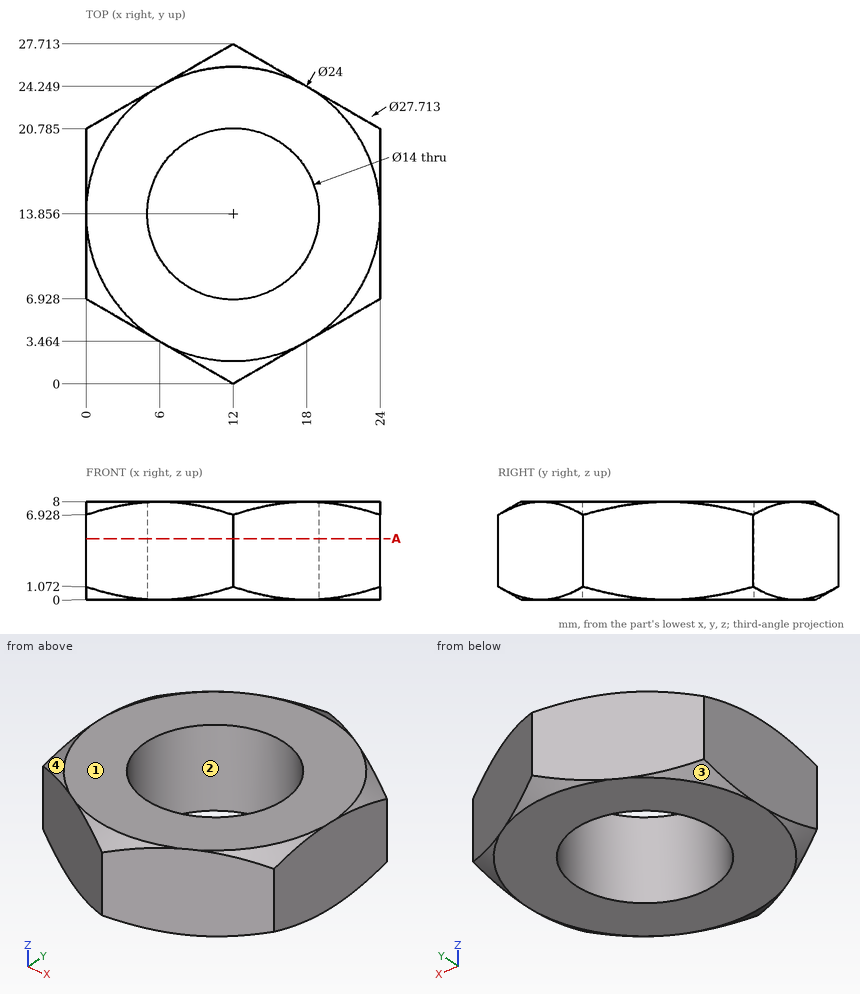
Answer from the drawing. Dimensions are ordinates in mm from the lowest x, y and z of the part. Give positions to 0.01 mm unless a question says otherwise; leave off trailing zeros. Write each loop counter-clockwise with the first axis right and the second up, starting at its lowest first coordinate (ties: lowest second). Pieces come first, ordered by that corner, then holes. Notation, with made-up numbers: (56.25, 0) -> (98.25, 0) arc R20 cw to (98.25, 22) -> close; hole circle Ø1 at (0.25, -6.75). An arc over 180 degrees is marked (long way). Use a Markdown table: item, result.
(1) Flat-ended cylindrical pins translate along their axes: P1, Ø1, axis at x = 21.5, z = 1.5, coming from the +Y side; P2, Ø1.5, axis at x = 14, z = 5, coming from the -Y side. Find the tip coordinate at first contact, or state that the pin passes through.
Return value:
| item | result |
|---|---|
| P1 | y = 22.52 |
| P2 | y = 0.72 |
(2) Find the intervals of material crossed by probe 1 along X at (y, z) = (18, 2); probe 2 along X at (y, z) = (9.25, 3.25); probe 3 along Y at (x, z) = (17, 2) (1 decimal), in increasing order. Write a range as from..to.
Return value:
| item | result |
|---|---|
| probe 1 | 0..6.36, 17.64..24 |
| probe 2 | 0..6.73, 17.27..24 |
| probe 3 | 2.9..9, 18.8..24.8 |
(3) Determine the mould class of the marked faces 1, 2, 3 and 4 for opening direction Y: released by +Y, released by -Y, zero draft, split by the parting line, or undercut.
Return value:
| item | result |
|---|---|
| face 1 | zero draft |
| face 2 | undercut |
| face 3 | released by +Y |
| face 4 | released by -Y |
(4) Section A-A, the plane z = 5 is taken. Determine the outline of the cut face in (x, y) (1 decimal).
Return value:
| item | result |
|---|---|
| outline | (0, 6.9) -> (12, 0) -> (24, 6.9) -> (24, 20.8) -> (12, 27.7) -> (0, 20.8) -> close; hole circle Ø14 at (12, 13.9) |
